```python
from build123d import *

# Parameters (mm, degrees)
CYLINDER018_R           = 1.75
CYLINDER018_DEPTH       = 68
CYLINDER018_PITCH_ANGLE = 90
SKETCH020_W             = 3
SKETCH020_H             = 13
PAD022_DEPTH            = 15
PAD020_DEPTH            = 6.1
CYLINDER002_R           = 1.75
CYLINDER002_DEPTH       = 30
CYLINDER003_R           = 1.75
CYLINDER003_DEPTH       = 30
CYLINDER001_R           = 1.75
CYLINDER001_DEPTH       = 30
CYLINDER_R              = 1.75
CYLINDER_DEPTH          = 30
BOX011_W                = 7
BOX011_H                = 6
BOX011_DEPTH            = 10
FILLET006_R             = 1
BOX008_W                = 32
BOX008_H                = 57
BOX008_DEPTH            = 27
SKETCH_R                = 1
SKETCH_W                = 13
SKETCH_H                = 23.5
PAD_DEPTH               = 40
BOX007_W                = 58
BOX007_H                = 68
BOX007_DEPTH            = 27
BOX001_W                = 62
BOX001_H                = 72
BOX001_DEPTH            = 26
FILLET007_R             = 1
CHAMFER_SIZE            = 1
FILLET008_R             = 1


with BuildPart() as cilindro:
    # Cylinder018 → Cylinder018 (new body)
    with BuildSketch(Plane.XY):
        Circle(CYLINDER018_R)
    extrude(amount=CYLINDER018_DEPTH)


with BuildPart() as cilindro_1:
    # Cylinder018 pitch: moved
    add(cilindro.part.rotate(Axis((0, 0, 0), (0, 1, 0)), CYLINDER018_PITCH_ANGLE))


with BuildPart() as cilindro_2:
    # Cylinder018 placement: moved
    add(cilindro_1.part.moved(Location((-34, 0, 18))))


with BuildPart() as cono:
    # Cone → Cone (revolve)
    with BuildSketch(Plane(origin=(-13, -31.5, -4), x_dir=(1, 0, 0), z_dir=(0, -1, 0))):
        Polygon((0, 0), (3.8, 0), (1, 3), (0, 3), align=None)
    revolve(axis=Axis((-13, -31.5, -4), (0, 0, 1)))


with BuildPart() as part_mirroring029:
    # Part__Mirroring029: instance of Cono
    add(cono.part.mirror(Plane(origin=(0, 0, 0), x_dir=(0, -1, 0), z_dir=(1, 0, 0))))


with BuildPart() as part_mirroring031:
    # Part__Mirroring031: instance of Part__Mirroring029
    add(part_mirroring029.part.mirror(Plane(origin=(0, 0, 0), x_dir=(1, 0, 0), z_dir=(0, 1, 0))))


with BuildPart() as fusion015:
    # Part__Mirroring030: instance of Cono
    add(cono.part.mirror(Plane(origin=(0, 0, 0), x_dir=(1, 0, 0), z_dir=(0, 1, 0))))

    # Fusion015: union Part__Mirroring031, Cono, Part__Mirroring029
    add(part_mirroring031.part)
    add(cono.part)
    add(part_mirroring029.part)


with BuildPart() as pad022:
    # Sketch020 → Pad022 (new body)
    with BuildSketch(Plane.XY.offset(10)):
        with Locations((-23, 0)):
            Rectangle(SKETCH020_W, SKETCH020_H)
        with Locations((23, 0)):
            Rectangle(SKETCH020_W, SKETCH020_H)
    extrude(amount=-PAD022_DEPTH)


with BuildPart() as pad020:
    # Sketch017 → Pad020 (new body)
    with BuildSketch(Plane(origin=(0, 40, 0), x_dir=(-1, 0, 0), z_dir=(0, 1, 0))):
        with BuildLine():
            Line((-7, 10), (7, 10))
            ThreePointArc((8.5, 8.5), (8.06066, 9.56066), (7, 10))
            Line((8.5, 8.5), (8.5, 4.5))
            ThreePointArc((7, 3), (8.06066, 3.43934), (8.5, 4.5))
            Line((7, 3), (-7, 3))
            ThreePointArc((-8.5, 4.5), (-8.06066, 3.43934), (-7, 3))
            Line((-8.5, 4.5), (-8.5, 8.5))
            ThreePointArc((-7, 10), (-8.06066, 9.56066), (-8.5, 8.5))
        make_face()
    extrude(amount=-PAD020_DEPTH)


with BuildPart() as cilindro002:
    # Cylinder002 → Cylinder002 (new body)
    with BuildSketch(Plane(origin=(-13, -31.5, -10), x_dir=(1, 0, 0), z_dir=(0, 0, 1))):
        Circle(CYLINDER002_R)
    extrude(amount=CYLINDER002_DEPTH)


with BuildPart() as cilindro003:
    # Cylinder003 → Cylinder003 (new body)
    with BuildSketch(Plane(origin=(13, -31.5, -10), x_dir=(1, 0, 0), z_dir=(0, 0, 1))):
        Circle(CYLINDER003_R)
    extrude(amount=CYLINDER003_DEPTH)


with BuildPart() as cilindro001:
    # Cylinder001 → Cylinder001 (new body)
    with BuildSketch(Plane(origin=(13, 31.5, -10), x_dir=(1, 0, 0), z_dir=(0, 0, 1))):
        Circle(CYLINDER001_R)
    extrude(amount=CYLINDER001_DEPTH)


with BuildPart() as fusion012:
    # Cylinder → Cylinder (new body)
    with BuildSketch(Plane(origin=(-13, 31.5, -10), x_dir=(1, 0, 0), z_dir=(0, 0, 1))):
        Circle(CYLINDER_R)
    extrude(amount=CYLINDER_DEPTH)

    # Fusion012: union Cilindro002, Cilindro003, Cilindro001
    add(cilindro002.part)
    add(cilindro003.part)
    add(cilindro001.part)


with BuildPart() as fillet006:
    # Box011 → Box011 (new body)
    with BuildSketch(Plane(origin=(-16, 28.5, 0), x_dir=(1, 0, 0), z_dir=(0, 0, 1))):
        with Locations((3.5, 3)):
            Rectangle(BOX011_W, BOX011_H)
    extrude(amount=BOX011_DEPTH)

    # Fillet006
    fillet006_edges = [fillet006.edges().sort_by_distance(p)[0] for p in [
        (-9, 28.5, 5),
    ]]
    fillet(fillet006_edges, radius=FILLET006_R)


with BuildPart() as part_mirroring027:
    # Part__Mirroring027: instance of Fillet006
    add(fillet006.part.mirror(Plane(origin=(0, 0, 0), x_dir=(1, 0, 0), z_dir=(0, 1, 0))))


with BuildPart() as part_mirroring026:
    # Part__Mirroring026: instance of Fillet006
    add(fillet006.part.mirror(Plane(origin=(0, 0, 0), x_dir=(0, -1, 0), z_dir=(1, 0, 0))))


with BuildPart() as part_mirroring028:
    # Part__Mirroring028: instance of Part__Mirroring026
    add(part_mirroring026.part.mirror(Plane(origin=(0, 0, 0), x_dir=(1, 0, 0), z_dir=(0, 1, 0))))


with BuildPart() as fusion013:
    # Fusion013 base: copy of Part__Mirroring026
    add(part_mirroring026.part)

    # Fusion013: union Fillet006, Part__Mirroring027, Part__Mirroring028
    add(fillet006.part)
    add(part_mirroring027.part)
    add(part_mirroring028.part)


with BuildPart() as fusion013_1:
    # Fusion013 placement: moved
    add(fusion013.part.moved(Location((0, 0, 1))))


with BuildPart() as cubo008:
    # Box008 → Box008 (new body)
    with BuildSketch(Plane(origin=(-16, -28.5, -2), x_dir=(1, 0, 0), z_dir=(0, 0, 1))):
        with Locations((16, 28.5)):
            Rectangle(BOX008_W, BOX008_H)
    extrude(amount=BOX008_DEPTH)


with BuildPart() as pad:
    # Sketch → Pad (new body)
    with BuildSketch(Plane(origin=(0, 0, -10), x_dir=(1, 0, 0), z_dir=(0, 0, -1))):
        with Locations((-26.75, 31.25)):
            Circle(SKETCH_R)
        with Locations((-19.25, 31.25)):
            Circle(SKETCH_R)
        with Locations((-26.75, 3.25)):
            Circle(SKETCH_R)
        with Locations((-19.25, 3.25)):
            Circle(SKETCH_R)
        with Locations((-26.75, -3.25)):
            Circle(SKETCH_R)
        with Locations((-19.25, -3.25)):
            Circle(SKETCH_R)
        with Locations((-26.75, -31.25)):
            Circle(SKETCH_R)
        with Locations((-19.25, -31.25)):
            Circle(SKETCH_R)
        with Locations((19.25, 31.25)):
            Circle(SKETCH_R)
        with Locations((26.75, 31.25)):
            Circle(SKETCH_R)
        with Locations((19.25, 3.25)):
            Circle(SKETCH_R)
        with Locations((26.75, 3.25)):
            Circle(SKETCH_R)
        with Locations((19.25, -3.25)):
            Circle(SKETCH_R)
        with Locations((26.75, -3.25)):
            Circle(SKETCH_R)
        with Locations((19.25, -31.25)):
            Circle(SKETCH_R)
        with Locations((26.75, -31.25)):
            Circle(SKETCH_R)
        with Locations((-23, 17.25)):
            Rectangle(SKETCH_W, SKETCH_H)
        with Locations((23, 17.25)):
            Rectangle(SKETCH_W, SKETCH_H)
        with Locations((-23, -17.25)):
            Rectangle(SKETCH_W, SKETCH_H)
        with Locations((23, -17.25)):
            Rectangle(SKETCH_W, SKETCH_H)
    extrude(amount=-PAD_DEPTH)


with BuildPart() as cubo007:
    # Box007 → Box007 (new body)
    with BuildSketch(Plane(origin=(-29, -34, 1.5), x_dir=(1, 0, 0), z_dir=(0, 0, 1))):
        with Locations((29, 34)):
            Rectangle(BOX007_W, BOX007_H)
    extrude(amount=BOX007_DEPTH)


with BuildPart() as obj1:
    # Box001 → Box001 (new body)
    with BuildSketch(Plane(origin=(-31, -36, -3.5), x_dir=(1, 0, 0), z_dir=(0, 0, 1))):
        with Locations((31, 36)):
            Rectangle(BOX001_W, BOX001_H)
    extrude(amount=BOX001_DEPTH)

    # Cut: cut Cubo007
    add(cubo007.part, mode=Mode.SUBTRACT)

    # Cut001: cut Pad
    add(pad.part, mode=Mode.SUBTRACT)

    # Cut002: cut Cubo008
    add(cubo008.part, mode=Mode.SUBTRACT)

    # Fusion014: union Fusion013
    add(fusion013_1.part)

    # Cut021: cut Fusion012
    add(fusion012.part, mode=Mode.SUBTRACT)

    # Cut022: cut Pad020
    add(pad020.part, mode=Mode.SUBTRACT)

    # Fillet007
    fillet007_edges = [obj1.edges().sort_by_distance(p)[0] for p in [
        (29, -34, 12),
        (29, 34, 12),
        (-29, 34, 12),
        (-29, -34, 12),
    ]]
    fillet(fillet007_edges, radius=FILLET007_R)

    # Chamfer
    chamfer_edges = [obj1.edges().sort_by_distance(p)[0] for p in [
        (-31, -36, 9.5),
        (-31, 36, 9.5),
        (-31, 0, -3.5),
        (0, 36, -3.5),
        (31, 36, 9.5),
        (0, -36, -3.5),
        (31, -36, 9.5),
        (31, 0, -3.5),
    ]]
    chamfer(chamfer_edges, length=CHAMFER_SIZE)

    # Cut024: cut Pad022
    add(pad022.part, mode=Mode.SUBTRACT)

    # Fillet008
    fillet008_edges = [obj1.edges().sort_by_distance(p)[0] for p in [
        (24.5, -5.5, -1),
        (24.5, 5.5, -1),
        (-24.5, -5.5, -1),
        (-24.5, 5.5, -1),
        (21.5, 5.5, -1),
        (21.5, -5.5, -1),
        (-21.5, -5.5, -1),
        (-21.5, 5.5, -1),
    ]]
    fillet(fillet008_edges, radius=FILLET008_R)

    # Cut025: cut Fusion015
    add(fusion015.part, mode=Mode.SUBTRACT)

    # Cut026: cut Cilindro
    add(cilindro_2.part, mode=Mode.SUBTRACT)


solid = obj1.part
```
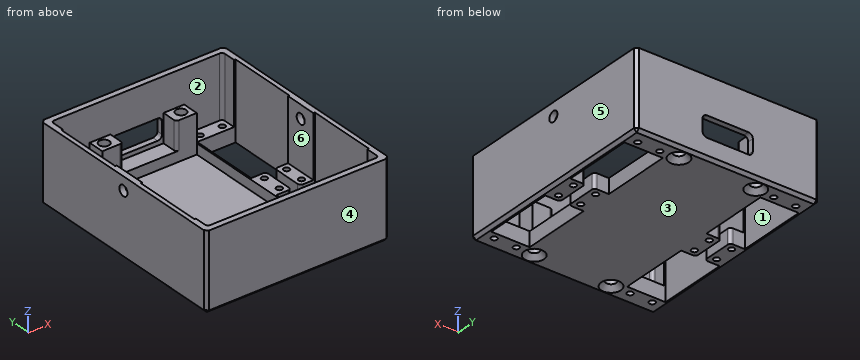
Work out the finished part from the listing and answer in its coordinate system (mm). Face numbers are marked on the shaded views. A direction names the side the tool comes from. Give positions to 0.01 mm unless a question says otherwise; leave off trailing zeros. Write each loop counter-clockwise with the first axis right and the second up, starting at its lowest first coordinate (ties: lowest second). Pieces come first, ordered by that corner, then holes. Notation, with made-up numbers: (17.5, -30.5) -> (35.5, -30.5) arc R15 ccw to (35.5, -26.5) -> close; hole circle Ø6 at (74, 22.25). An arc over 180 degrees is marked (long way). Write item = value, one per line.
Q1. Flat-ended cylindrical pins translate along their axes: pin 1 Ø10 at (x, y) = (-2.5, 10) entering from +Z; pin 2 Ø4.5 at (x, y) = (13, -31.5) entering from -Z; pin 3 Ø3 at (x, y) = (12, 31.5) entering from +Z; pin 4 Ø1.2 at (x, y) = (19.25, 31.25) entering from +Z. Find the tip coordinate at first contact, or state that the pin passes through.
Computed values:
pin_1 = -2
pin_2 = -2.34
pin_3 = 11
pin_4 = through
Q2. Section C-C on x = 13 is taken. Determine the outline of the cut face in (y, z), and give its area (3 significant figures).
Computed values:
outline = (-36, -2.5) -> (-35, -3.5) -> (-34.83, -3.5) -> (-33.25, -1.8) -> (-33.25, 11) -> (-34, 11) -> (-34, 22.5) -> (-36, 22.5) -> close; (-29.75, -1.8) -> (-28.17, -3.5) -> (28.17, -3.5) -> (29.75, -1.8) -> (29.75, 11) -> (28.5, 11) -> (28.5, -2) -> (-28.5, -2) -> (-28.5, 11) -> (-29.75, 11) -> close; (33.25, -1.8) -> (34.83, -3.5) -> (35, -3.5) -> (36, -2.5) -> (36, 22.5) -> (34, 22.5) -> (34, 11) -> (33.25, 11) -> close
area = 241 mm^2
Q3. For a pull along X with two mould halves and no side action, classify the marked faces 4, 5 and 6 as pulls with the +X half, pulls with the -X half, needs draft (parallel to the pull), parting line crosses it, or undercut.
Computed values:
face_4 = needs draft
face_5 = pulls with the +X half
face_6 = undercut
Q4. Section A-A on x = -19.25 is taken. State how many separate pieces and enclosed holes the cut face has, and give its area (3 significant figures).
Computed values:
separate_pieces = 7
enclosed_holes = 0
area = 168 mm^2
Q5. Section D-D on y = -17.5 is taken. Determine the outline of the cut face in (x, z).
Computed values:
outline = (-31, -2.5) -> (-30, -3.5) -> (-29.5, -3.5) -> (-29.5, 22.5) -> (-31, 22.5) -> close; (-16.5, -3.5) -> (16.5, -3.5) -> (16.5, 1.5) -> (16, 1.5) -> (16, -2) -> (-16, -2) -> (-16, 1.5) -> (-16.5, 1.5) -> close; (29.5, -3.5) -> (30, -3.5) -> (31, -2.5) -> (31, 22.5) -> (29.5, 22.5) -> close
Q6. A tool of negligible diameter and unlimited length cuts with its end or side. For the marked faces 1, 2 and 3, from which of +Z, -Z, +X, -X, +Y, -Y can it reach the whole face along a straight path? Write none if from no direction.
Computed values:
face_1 = +Z, -Z
face_2 = +Z
face_3 = -Z, +X, -X, +Y, -Y
Q7. Consider line 1 along X through (y, z) = (-24, -1.5); line 2 along X through (y, z) = (-31.5, 6); line 3 along X through (y, z) = (-0.5, 2.5). Determine where each line is inside the solid, lowest interval first.
Computed values:
line_1 = -31 to -29.5, -16.5 to -16, 16 to 16.5, 29.5 to 31
line_2 = -31 to -29, -16 to -14.75, -11.25 to -9, 9 to 11.25, 14.75 to 16, 29 to 31
line_3 = -31 to -29, 29 to 31
